The listing builds one solid part. Answer for the finished solid, in the listing's coordinates (mm). Face numbers are marked on the shaded views. A direction names the side the tool comes from. Coordinates: 2 decimals unless noted, no trailing zeros. Write each loop counter-clockwise with the first axis right and the second up, starting at its lowest first coordinate (ties: lowest second). Pieces come first, ordered by that corner, then holes.
from build123d import *

# Parameters (mm, degrees)
SKETCH1_R           = 62.5
SKETCH1_R_2         = 52.5
BOSS_EXTRUDE1_DEPTH = 10
BOSS_EXTRUDE5_DEPTH = 10
CUT_EXTRUDE2_DEPTH  = 7.25
SKETCH4_R           = 1.875
CUT_EXTRUDE3_DEPTH  = 6
SKETCH5_R           = 1.75
CUT_EXTRUDE4_DEPTH  = 5
FILLET1_R           = 2.5
CHAMFER1_SIZE       = 1.25


with BuildPart() as part:
    # Sketch1 → Boss-Extrude1 (new body)
    with BuildSketch(Plane.XY):
        Circle(SKETCH1_R)
        Circle(SKETCH1_R_2, mode=Mode.SUBTRACT)
    extrude(amount=-BOSS_EXTRUDE1_DEPTH)

    # Sketch2 → Boss-Extrude5 (add)
    with BuildSketch(Plane.XY):
        with BuildLine():
            Line((46.892042254, -23.609031603), (9.761355821, -2.171619796))
            ThreePointArc((9.761355821, -2.171619796), (8.660254038, 5), (3, 9.539392014))
            Line((3, 9.539392014), (3, 52.414215629))
            ThreePointArc((3, 52.414215629), (0, 52.5), (-3, 52.414215629))
            Line((-3, 52.414215629), (-3, 9.539392014))
            ThreePointArc((-3, 9.539392014), (-8.660254038, 5), (-9.761355821, -2.171619796))
            Line((-9.761355821, -2.171619796), (-46.892042254, -23.609031603))
            ThreePointArc((-46.892042254, -23.609031603), (-45.466333699, -26.25), (-43.892042254, -28.805184026))
            Line((-43.892042254, -28.805184026), (-6.761355821, -7.367772218))
            ThreePointArc((-6.761355821, -7.367772218), (0, -10), (6.761355821, -7.367772218))
            Line((6.761355821, -7.367772218), (43.892042254, -28.805184026))
            ThreePointArc((43.892042254, -28.805184026), (45.466333699, -26.25), (46.892042254, -23.609031603))
        make_face()
    extrude(amount=-BOSS_EXTRUDE5_DEPTH)

    # Sketch3 → Cut-Extrude2 (cut)
    with BuildSketch(Plane.XY.offset(-10)):
        Polygon((0, 6), (-5.196152423, 3), (-5.196152423, -3), (0, -6), (5.196152423, -3), (5.196152423, 3), align=None)
    extrude(amount=CUT_EXTRUDE2_DEPTH, mode=Mode.SUBTRACT)

    # Sketch4 → Cut-Extrude3 (cut)
    with BuildSketch(Plane.XY):
        Circle(SKETCH4_R)
    extrude(amount=-CUT_EXTRUDE3_DEPTH, mode=Mode.SUBTRACT)

    # Sketch5 → Cut-Extrude4 (cut)
    with BuildSketch(Plane.XY):
        with Locations((12.794953702, 56.05835495)):
            Circle(SKETCH5_R)
        with Locations((0, 57.5)):
            Circle(SKETCH5_R)
        with Locations((24.948314999, 51.805709904)):
            Circle(SKETCH5_R)
        with Locations((35.850663607, 44.955310242)):
            Circle(SKETCH5_R)
        with Locations((44.955310242, 35.850663607)):
            Circle(SKETCH5_R)
        with Locations((51.805709904, 24.948314999)):
            Circle(SKETCH5_R)
        with Locations((56.05835495, 12.794953702)):
            Circle(SKETCH5_R)
        with Locations((57.5, 0)):
            Circle(SKETCH5_R)
        with Locations((56.05835495, -12.794953702)):
            Circle(SKETCH5_R)
        with Locations((51.805709904, -24.948314999)):
            Circle(SKETCH5_R)
        with Locations((44.955310242, -35.850663607)):
            Circle(SKETCH5_R)
        with Locations((35.850663607, -44.955310242)):
            Circle(SKETCH5_R)
        with Locations((24.948314999, -51.805709904)):
            Circle(SKETCH5_R)
        with Locations((12.794953702, -56.05835495)):
            Circle(SKETCH5_R)
        with Locations((0, -57.5)):
            Circle(SKETCH5_R)
        with Locations((-12.794953702, -56.05835495)):
            Circle(SKETCH5_R)
        with Locations((-24.948314999, -51.805709904)):
            Circle(SKETCH5_R)
        with Locations((-35.850663607, -44.955310242)):
            Circle(SKETCH5_R)
        with Locations((-44.955310242, -35.850663607)):
            Circle(SKETCH5_R)
        with Locations((-51.805709904, -24.948314999)):
            Circle(SKETCH5_R)
        with Locations((-56.05835495, -12.794953702)):
            Circle(SKETCH5_R)
        with Locations((-57.5, 0)):
            Circle(SKETCH5_R)
        with Locations((-56.05835495, 12.794953702)):
            Circle(SKETCH5_R)
        with Locations((-51.805709904, 24.948314999)):
            Circle(SKETCH5_R)
        with Locations((-44.955310242, 35.850663607)):
            Circle(SKETCH5_R)
        with Locations((-35.850663607, 44.955310242)):
            Circle(SKETCH5_R)
        with Locations((-24.948314999, 51.805709904)):
            Circle(SKETCH5_R)
        with Locations((-12.794953702, 56.05835495)):
            Circle(SKETCH5_R)
    extrude(amount=-CUT_EXTRUDE4_DEPTH, mode=Mode.SUBTRACT)

    # Fillet1
    fillet1_edges = [part.edges().sort_by_distance(p)[0] for p in [
        (3, 52.414215629, -5),
        (46.892042254, -23.609031603, -5),
        (43.892042254, -28.805184026, -5),
        (-43.892042254, -28.805184026, -5),
        (-46.892042254, -23.609031603, -5),
        (-3, 52.414215629, -5),
    ]]
    fillet(fillet1_edges, radius=FILLET1_R)

    # Chamfer1
    chamfer1_edges = [part.edges().sort_by_distance(p)[0] for p in [
        (3, 29.617985687, -10),
        (27.149928014, -12.210916632, 0),
        (24.149928014, -17.407069055, -10),
        (-24.149928014, -17.407069055, 0),
        (-27.149928014, -12.210916632, -10),
        (-3, 29.617985687, 0),
        (-62.5, 0, 0),
        (27.149928014, -12.210916632, -10),
        (-24.149928014, -17.407069055, -10),
        (-3, 29.617985687, -10),
        (3, 29.617985687, 0),
        (-8.660254038, 5, 0),
        (-27.149928014, -12.210916632, 0),
        (0, -10, 0),
        (24.149928014, -17.407069055, 0),
        (45.466333699, 26.25, 0),
        (45.466333699, 26.25, -10),
        (8.660254038, 5, 0),
        (0, -52.5, 0),
        (0, -52.5, -10),
        (-45.466333699, 26.25, 0),
        (-45.466333699, 26.25, -10),
        (46.56758219, -22.460656486, 0),
        (46.56758219, -22.460656486, -10),
        (42.735290198, -29.098380926, 0),
        (42.735290198, -29.098380926, -10),
        (-42.735290198, -29.098380926, 0),
        (-42.735290198, -29.098380926, -10),
        (-46.56758219, -22.460656486, 0),
        (-46.56758219, -22.460656486, -10),
        (3.832291992, 51.559037412, 0),
        (3.832291992, 51.559037412, -10),
        (-3.832291992, 51.559037412, 0),
        (-3.832291992, 51.559037412, -10),
        (-62.5, 0, -10),
    ]]
    chamfer(chamfer1_edges, length=CHAMFER1_SIZE)


solid = part.part
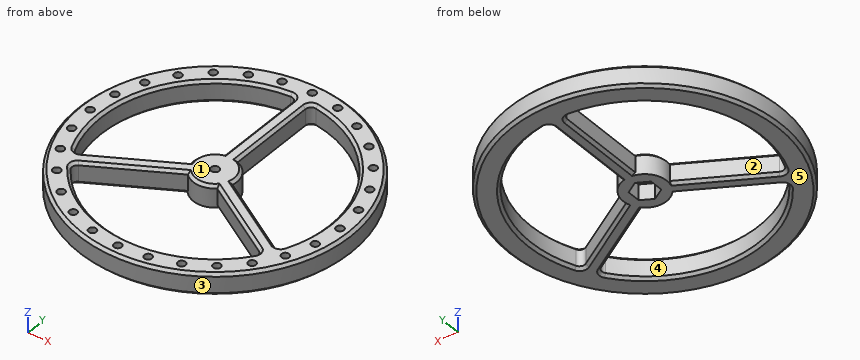
1. For a pull along X with two mould halves and no side action, classify the marked faces 3, 4 and 5 as pulls with the +X half, pulls with the -X half, needs draft (parallel to the pull), parting line crosses it, or undercut.
Results found:
face 3: parting line crosses it
face 4: undercut
face 5: needs draft
2. Flat-ended cylindrical pins translate along their axes: P1, Ø3, axis at x = -0.5, y = 1, coming from the -Z side; P2, Ø5, axis at x = -46.5, y = -15.5, coming from the +Z side; P3, Ø6, axis at y = -40, z = -6.5, coming from the +X side; P4, Ø6, axis at x = 14, z = -5, coming from the +Y side. Find the tip coordinate at first contact, or state that the pin passes through.
Results found:
P1: stops at z = -2.75
P2: passes through
P3: stops at x = 50.37
P4: stops at y = 61.52
3. Section B-B on y = 0 is taken. State how many separate pieces and enclosed holes the cut face has, then the cut area to 3 significant figures.
Results found:
separate pieces: 4
enclosed holes: 0
area: 272 mm2
4. Find the intervals of material crossed by L1, parallel to X at y = 40, z = -5.25; L2, parallel to X at y = -1, z = -8.25; L3, parallel to X at y = 33.5, z = -6, in increasing order.
Results found:
L1: x = -48.02 to -34, -3 to 3, 34 to 48.02
L2: x = -62.49 to -52.49, -9.95 to -5.2, 5.2 to 9.95, 52.49 to 62.49
L3: x = -52.76 to -40.42, -3 to 3, 40.42 to 52.76
5. Section A-A on z = -7 is taken. Give the vertices of the cut face in (x, y) (1 decimal), then the cut area to 3 significant figures.
Results found:
outline: circle Ø125 at (0, 0); hole (-48.1, -21.1) arc R2.5 ccw to (-44.5, -22.3) - (-9.8, -2.2) arc R10 cw to (-3, 9.5) - (-3, 49.7) arc R2.5 ccw to (-5.8, 52.2) arc R52.5 ccw to start; hole (-42.3, -31.1) arc R52.5 ccw to (42.3, -31.1) arc R2.5 ccw to (41.5, -27.4) - (6.8, -7.4) arc R10 cw to (-6.8, -7.4) - (-41.5, -27.4) arc R2.5 ccw to start; hole (-5.2, -3) - (0, -6) - (5.2, -3) - (5.2, 3) - (0, 6) - (-5.2, 3) - close; hole (3, 9.5) arc R10 cw to (9.8, -2.2) - (44.5, -22.3) arc R2.5 ccw to (48.1, -21.1) arc R52.5 ccw to (5.8, 52.2) arc R2.5 ccw to (3, 49.7) - close
area: 4,610 mm2
6. A tool of negligible diameter and unlimited length cuts with its end or side. For the marked faces 1 and 2, from which of +Z, -Z, +X, -X, +Y, -Y can it reach the whole face along a straight path? Write none if from no direction.
Results found:
face 1: +Z, +X, -X, +Y, -Y
face 2: +Z, -Z
